from build123d import *

# Parameters (mm, degrees)
ESBO_O1_R                = 3.175
ESBO_O1_R_2              = 3.6
ESBO_O1_R_3              = 4.4
RESSALTO_EXTRUS_O1_DEPTH = 12.7
ESBO_O3_R                = 5.85
CORTE_EXTRUS_O1_DEPTH    = 1


with BuildPart() as part:
    # Esboço1 → Ressalto-extrusão1 (new body)
    with BuildSketch(Plane.XY):
        with BuildLine():
            Line((68.264029726, 80.471482556), (86.913718709, 78.564915838))
            ThreePointArc((86.913718709, 78.564915838), (96.190192778, 50.934582064), (123.199407881, 39.98055928))
            ThreePointArc((123.199407881, 39.98055928), (126.9879217, 39.943074462), (130.568554452, 38.704805036))
            ThreePointArc((130.568554452, 38.704805036), (112.191596118, 24.182863465), (91.421685961, 13.356496733))
            ThreePointArc((91.421685961, 13.356496733), (70.502377652, 7.424980082), (48.785297914, 8.506089469))
            ThreePointArc((48.785297914, 8.506089469), (29.282001901, 15.926871282), (17.091631159, 32.863264618))
            ThreePointArc((17.091631159, 32.863264618), (12.862793068, 38.519278229), (7.740980224, 43.381437705))
            Line((7.740980224, 43.381437705), (18.663600862, 58.560101484))
            ThreePointArc((18.663600862, 58.560101484), (49.782513053, 55.212261005), (68.264029726, 80.471482556))
        make_face()
        with Locations((72.07343938, 70.420125946)):
            Circle(ESBO_O1_R, mode=Mode.SUBTRACT)
        with Locations((23.31829005, 48.678964138)):
            Circle(ESBO_O1_R_2, mode=Mode.SUBTRACT)
        with Locations((35.486495683, 29.988548249)):
            Circle(ESBO_O1_R_2, mode=Mode.SUBTRACT)
        with Locations((105.243732184, 30.464144141)):
            Circle(ESBO_O1_R_2, mode=Mode.SUBTRACT)
        with Locations((52.234302046, 49.457669457)):
            Circle(ESBO_O1_R_3, mode=Mode.SUBTRACT)
    extrude(amount=RESSALTO_EXTRUS_O1_DEPTH)

    # Esboço3 → Corte-extrusão1 (cut)
    with BuildSketch(Plane.XY.offset(12.7)):
        with Locations((52.234302046, 49.457669457)):
            Circle(ESBO_O3_R)
    extrude(amount=-CORTE_EXTRUS_O1_DEPTH, mode=Mode.SUBTRACT)


solid = part.part
Build history of the part. All positions in model axes, mm. A direction names the side the tool comes from. Coordinates: 2 decimals unless noted, no trailing zeros. Order: outer loops, then holes, each group sorted by start corner. A loop starts at its lowest first (then second) coordinate and runs counter-clockwise, first axis right, second up. Notation, with made-up numbers: (81, 2) - (87, 2) arc R23 ccw to (87, 26) - close; hole circle Ø10 at (31.25, -23). An arc over 180 degrees is marked (long way). Write item = value, one per line. Start each with the question number.
1) Saw through at D-D on x = 70.5. Write the cut outline in (y, z), then the cut area to 3 significant figures.
2) Saw through at B-B on y = 47. Write the cut outline in (x, z).
3) Wall check: line 1 along X through (y, z) = (52, 5.5); line 2 along X through (y, z) = (31, 6.5); line 3 along Y through (x, z) = (34, 6.5). Give the ranges that are in metal, low to high. Write a range as from..to.
4) 3-axis set-ups, long thin cutter, end or side, ignore diameter. For faces 1 (the face through (34.706, 26.474, 6.261)), 2 (the face through (53, 54, 11.7)): which of +Z, -Z, +X, -X, +Y, -Y reach the whole face in a straight line?
5) Flat gauge pins, fed straight in: pin 1 Ø6 at (y, z) = (67.5, 8.5) entering from -X; pin 2 Ø11.5 at (x, y) = (52.23, 49.46) entering from +Z; pin 3 Ø5 at (x, z) = (97.5, 2.5) entering from -Y. Where does each tip first touch, or does it go through?
6) Two-plate mould, pull along Y, no slides. Class faces 3 (the face through (70, 36, 12.7)), 4 (the face through (77.46, 79.53, 6.26)), 5 (the face through (69.55, 68.49, 6.26)): pulls with the +Y half, pulls with the -Y half, needs draft (parallel to the pull), parting line crosses it, or undercut.
7) Saw through at A-A on x = 103. Write the cut outline in (y, z), then the cut area to 3 significant figures.
8) Saw through at C-C on z = 4.75. Count the separate pieces of the cut face and the enclosed holes in it, then the cut area to 3 significant figures.
From the geometry:
q1.outline = (7.42, 0) - (67.66, 0) - (67.66, 12.7) - (7.42, 12.7) - close; (73.18, 0) - (80.24, 0) - (80.24, 12.7) - (73.18, 12.7) - close
q1.area = 855 mm^2
q2.outline = (10.34, 0) - (20.13, 0) - (20.13, 12.7) - (10.34, 12.7) - close; (26.5, 0) - (48.58, 0) - (48.58, 11.7) - (46.93, 11.7) - (46.93, 12.7) - (26.5, 12.7) - close; (55.88, 0) - (100.57, 0) - (100.57, 12.7) - (57.54, 12.7) - (57.54, 11.7) - (55.88, 11.7) - close
q3.line_1 = 13.94..21.93, 24.71..48.64, 55.83..95.23
q3.line_2 = 17.79..32.03, 38.94..101.68, 108.8..121.71
q3.line_3 = 12.85..26.71, 33.27..52.7
q4.face_1 = +Z, -Z
q4.face_2 = +Z
q5.pin_1 = 61.75
q5.pin_2 = 11.7
q5.pin_3 = 14.88
q6.face_3 = needs draft
q6.face_4 = pulls with the +Y half
q6.face_5 = undercut
q7.outline = (18.77, 0) - (27.65, 0) - (27.65, 12.7) - (18.77, 12.7) - close; (33.28, 0) - (45.32, 0) - (45.32, 12.7) - (33.28, 12.7) - close
q7.area = 266 mm^2
q8.separate_pieces = 1
q8.enclosed_holes = 5
q8.area = 4,500 mm^2
